Part print with two shaded views. Sizes in mm from the minimum x, y, z corner. A direction names the side the tool comes from. Give positions to 0.01 mm unless a question says otherwise; leave off trailing zeros. Write each loop counter-clockwise with the first axis right and the second up, starting at its lowest first coordinate (ties: lowest second). Pieces come first, ordered by that corner, then holes. Notation, with made-up numbers: M 3.25,79 L 40.25,79 A33 ccw 40.25,107 Z; hole C -32.5,-4 d3. An arc over 180 degrees is marked long. Return JSON: item names as keys, results as strings. Group by question number.
Q1. Tool access for the marked faces 4 and 5: list every direction of +Z, -Z, +X, -X, +Y, -Y with a clear straight run to the whole face (end or side of a thin tool).
Q2. Band-saw the part on C-C, the plane x = 64. Give the cut face in (y, z), then the cut area to 3 significant figures.
Q3. Pull direction Z, two halves, no side cores. Call the marked faces 1, 2 and 3: +Z half, -Z half, draft (parallel to the pull), parting line (faces both ways), or undercut.
Q4. Wall check: probe 1 along Z at (x, y) = (7.5, 9.25); probe 2 along Y at (x, z) = (50, 4.1). Give the ranges that are in metal, low to high.
Q5. Band-saw the part on B-B, the plane z = 71. Give the cut face in (x, y), then the cut area to 3 significant figures.
Q6. Band-saw the part on A-A, the plane y = 15. Give the cut face in (x, z), then the cut area to 3 significant figures.
Q7. Band-saw the part on D-D, the plane y = 3. Give the cut face in (x, z).
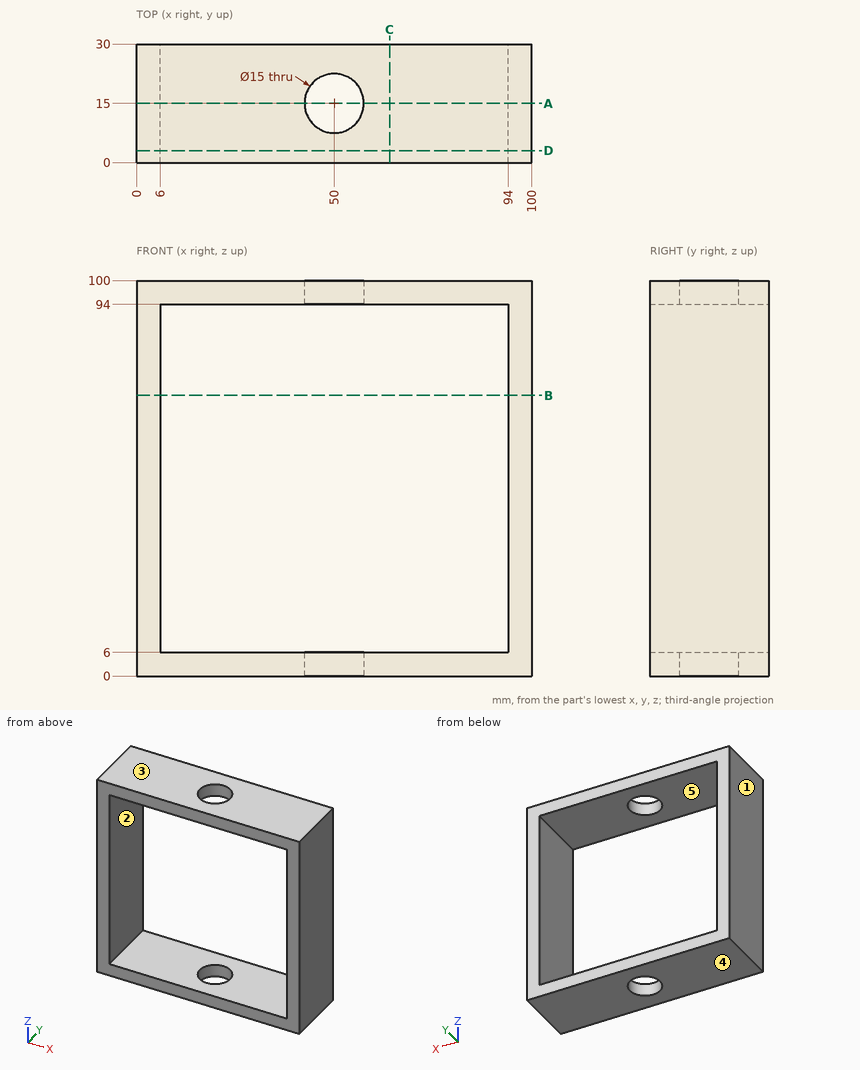
From the geometry:
{
 "1": {"face 4": "-Z, +X, -X, +Y, -Y", "face 5": "+Y, -Y"},
 "2": {"outline": "M 0,0 L 30,0 L 30,6 L 0,6 Z; M 0,94 L 30,94 L 30,100 L 0,100 Z", "area": "360 mm^2"},
 "3": {"face 1": "draft", "face 2": "undercut", "face 3": "+Z half"},
 "4": {"probe 1": "z = 0 to 6, 94 to 100", "probe 2": "y = 0 to 7.5, 22.5 to 30"},
 "5": {"outline": "M 0,0 L 6,0 L 6,30 L 0,30 Z; M 94,0 L 100,0 L 100,30 L 94,30 Z", "area": "360 mm^2"},
 "6": {"outline": "M 0,0 L 42.5,0 L 42.5,6 L 6,6 L 6,94 L 42.5,94 L 42.5,100 L 0,100 Z; M 57.5,0 L 100,0 L 100,100 L 57.5,100 L 57.5,94 L 94,94 L 94,6 L 57.5,6 Z", "area": "2,080 mm^2"},
 "7": {"outline": "M 0,0 L 100,0 L 100,100 L 0,100 Z; hole M 6,6 L 94,6 L 94,94 L 6,94 Z"}
}
